```python
from build123d import *

# Parameters (mm, degrees)
SKETCH1_W           = 114.3
SKETCH1_H           = 63.5
BOSS_EXTRUDE1_DEPTH = 3.175
SKETCH2_W           = 114.3
SKETCH2_H           = 63.5
SKETCH2_W_2         = 107.95
SKETCH2_H_2         = 57.15
BOSS_EXTRUDE2_DEPTH = 12.7
CUT_EXTRUDE1_REACH  = 121.685
SKETCH3_W           = 12.7
SKETCH3_H           = 12.7
SKETCH3_H_2         = 20.32
CUT_EXTRUDE2_REACH  = 68.599
SKETCH4_R           = 3.175


with BuildPart() as part:
    # Sketch1 → Boss-Extrude1 (new body)
    with BuildSketch(Plane.XY):
        Rectangle(SKETCH1_W, SKETCH1_H)
    extrude(amount=BOSS_EXTRUDE1_DEPTH)

    # Sketch2 → Boss-Extrude2 (add)
    with BuildSketch(Plane.XY.offset(3.175)):
        Rectangle(SKETCH2_W, SKETCH2_H)
        Rectangle(SKETCH2_W_2, SKETCH2_H_2, mode=Mode.SUBTRACT)
    extrude(amount=BOSS_EXTRUDE2_DEPTH)

    # Sketch3 → Cut-Extrude1 (cut, up to next)
    with BuildSketch(Plane.ZY.offset(57.15), mode=Mode.PRIVATE) as cut_extrude1_sk1:
        with Locations((9.525, -22.225)):
            Rectangle(SKETCH3_W, SKETCH3_H)
    cut_extrude1_tool1 = extrude(cut_extrude1_sk1.sketch, amount=-CUT_EXTRUDE1_REACH, mode=Mode.PRIVATE) & part.part
    # Sketch3 → Cut-Extrude1 (cut, up to next)
    with BuildSketch(Plane.ZY.offset(57.15), mode=Mode.PRIVATE) as cut_extrude1_sk2:
        with Locations((9.525, 18.415)):
            Rectangle(SKETCH3_W, SKETCH3_H_2)
    cut_extrude1_tool2 = extrude(cut_extrude1_sk2.sketch, amount=-CUT_EXTRUDE1_REACH, mode=Mode.PRIVATE) & part.part
    add(cut_extrude1_tool1.solids().sort_by_distance((-57.15, -22.225, 9.525))[0], mode=Mode.SUBTRACT)
    add(cut_extrude1_tool2.solids().sort_by_distance((-57.15, 18.415, 9.525))[0], mode=Mode.SUBTRACT)

    # Sketch4 → Cut-Extrude2 (cut, up to next)
    with BuildSketch(Plane.XY.offset(3.175), mode=Mode.PRIVATE) as cut_extrude2_sk1:
        with Locations((-44.45, 0)):
            Circle(SKETCH4_R)
    cut_extrude2_tool1 = extrude(cut_extrude2_sk1.sketch, amount=-CUT_EXTRUDE2_REACH, mode=Mode.PRIVATE) & part.part
    # Sketch4 → Cut-Extrude2 (cut, up to next)
    with BuildSketch(Plane.XY.offset(3.175), mode=Mode.PRIVATE) as cut_extrude2_sk2:
        with Locations((44.45, 0)):
            Circle(SKETCH4_R)
    cut_extrude2_tool2 = extrude(cut_extrude2_sk2.sketch, amount=-CUT_EXTRUDE2_REACH, mode=Mode.PRIVATE) & part.part
    add(cut_extrude2_tool1.solids().sort_by_distance((-44.45, 0, 3.175))[0], mode=Mode.SUBTRACT)
    add(cut_extrude2_tool2.solids().sort_by_distance((44.45, 0, 3.175))[0], mode=Mode.SUBTRACT)


solid = part.part
```
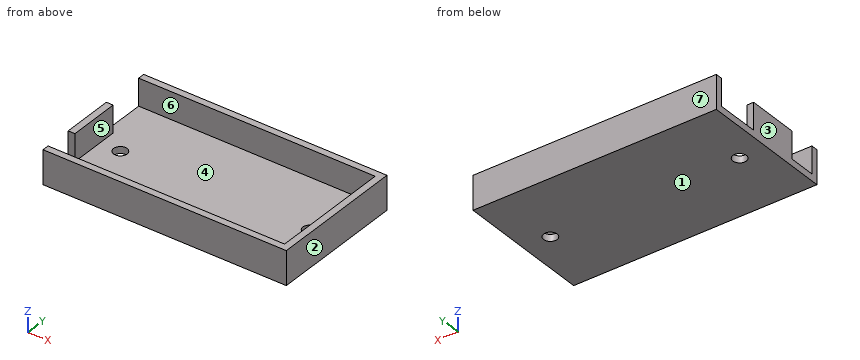
Design review of the part built by this model. Coordinates are the model's own, in mm. Face numbers are marked on the shaded views. A direction names the side the tool comes from. Round coordinates to 2 decimals unless told otherwise and drop trailing zeros. Write each loop counter-clockwise with the first axis right and the second up, starting at its lowest first coordinate (ties: lowest second). Pieces come first, ordered by that corner, then holes. Notation, with made-up numbers: (-28.5, 32.5) -> (26.5, 32.5) arc R19 cw to (26.5, 40.5) -> close; hole circle Ø10 at (71, 28.25). An arc over 180 degrees is marked (long way). Answer in a Markdown table with one row per item.
Q1. Clearance check with flat-ended pins moving along their axes: pin 1 Ø8.5 at (x, y) = (-44.45, 0) entering from +Z (3 decimals); pin 2 Ø4 at (x, y) = (44.45, 0) entering from -Z; pin 3 Ø8 at (y, z) = (23, 6) entering from -X. State where each tip first meets the part, or that it passes through.
The answers:
| item | result |
|---|---|
| pin 1 | z = 3.175 |
| pin 2 | through |
| pin 3 | x = -57.15 |
Q2. Take a section at D-D, the plane y = -10. State the section outline as (x, z) points (3 decimals), then the cut area to 3 significant figures.
The answers:
| item | result |
|---|---|
| outline | (-57.15, 0) -> (57.15, 0) -> (57.15, 15.875) -> (53.975, 15.875) -> (53.975, 3.175) -> (-53.975, 3.175) -> (-53.975, 15.875) -> (-57.15, 15.875) -> close |
| area | 444 mm² |
Q3. Take a section at C-C, the plane x = 44.45. State the section outline as (y, z) points (3 decimals), then the cut area to 3 significant figures.
The answers:
| item | result |
|---|---|
| outline | (-31.75, 0) -> (-3.175, 0) -> (-3.175, 3.175) -> (-28.575, 3.175) -> (-28.575, 15.875) -> (-31.75, 15.875) -> close; (3.175, 0) -> (31.75, 0) -> (31.75, 15.875) -> (28.575, 15.875) -> (28.575, 3.175) -> (3.175, 3.175) -> close |
| area | 262 mm² |
Q4. For the marked faces 5, 6 and 7, list the 3-axis set-ups (+Z, -Z, +X, -X, +Y, -Y) from which the entire face can be reached by the end or side of a thin tool; tool diameter is ignored.
The answers:
| item | result |
|---|---|
| face 5 | +Z |
| face 6 | +Z, -X |
| face 7 | +Z, -Z, +X, -X, +Y |
Q5. Take a section at A-A, the plane z = 12.25. State the section outline as (x, y) points (3 decimals).
The answers:
| item | result |
|---|---|
| outline | (-57.15, -31.75) -> (57.15, -31.75) -> (57.15, 31.75) -> (-57.15, 31.75) -> (-57.15, 28.575) -> (53.975, 28.575) -> (53.975, -28.575) -> (-57.15, -28.575) -> close; (-57.15, -15.875) -> (-53.975, -15.875) -> (-53.975, 8.255) -> (-57.15, 8.255) -> close |
Q6. Take a section at B-B, the plane y = 0. State the section outline as (x, z) points (3 decimals).
The answers:
| item | result |
|---|---|
| outline | (-57.15, 0) -> (-47.625, 0) -> (-47.625, 3.175) -> (-53.975, 3.175) -> (-53.975, 15.875) -> (-57.15, 15.875) -> close; (-41.275, 0) -> (41.275, 0) -> (41.275, 3.175) -> (-41.275, 3.175) -> close; (47.625, 0) -> (57.15, 0) -> (57.15, 15.875) -> (53.975, 15.875) -> (53.975, 3.175) -> (47.625, 3.175) -> close |
Q7. To check wall thickness, follow L1, parallel to Y at x = 13.5, z = 9.5 (3 decimals); L2, parallel to Y at x = 44.45, z = 1 (3 decimals); L3, parallel to X at y = 2, z = 10.75 (3 decimals). State the ranges of each line that lie inside material, in increasing order. Write a range as [from, to].
The answers:
| item | result |
|---|---|
| L1 | [-31.75, -28.575], [28.575, 31.75] |
| L2 | [-31.75, -3.175], [3.175, 31.75] |
| L3 | [-57.15, -53.975], [53.975, 57.15] |
Q8. Draft analysis for pull direction X (two halves, no side actions). For the marked faces 1, 2, 3 and 4, state which applies: +X half, -X half, draft (parallel to the pull), parting line (faces both ways), or undercut.
The answers:
| item | result |
|---|---|
| face 1 | draft |
| face 2 | +X half |
| face 3 | -X half |
| face 4 | undercut |
